CAD build for the part. Positions are in the model's coordinates, mm. A direction names the side the tool comes from. Round coordinates to 2 decimals unless told otherwise and drop trailing zeros. Order: outer loops, then holes, each group sorted by start corner. A loop starts at its lowest first (then second) coordinate and runs counter-clockwise, first axis right, second up. Notation, with made-up numbers: (-25.75, 42.5) - (23.25, 42.5) arc R29 cw to (23.25, 62.5) - close; hole circle Ø2 at (-14.75, 84). An arc over 180 degrees is marked (long way). Write item = value, one per line.
Autodesk Fusion 360 part; units mm, degrees
sketch "Sketch1" plane through (0, 0, 0) normal (0, 0, 1) x (1, 0, 0)
  circle A0 centre (0, 0) radius 115
  circle A1 centre (0, 0) radius 87.5 construction
  circle A2 centre (0, 0) radius 65
  circle A3 centre (0, 0) radius 50
  dimension "d1" = 230
  dimension "d2" = 175
  dimension "d3" = 130
  dimension "d4" = 100
extrude "Extrude1" add sketch "Sketch1" along normal blind 15 contours A0
extrude "Extrude2" add sketch "Sketch1" along normal blind 80 contours A2
sketch "Sketch2" plane through (0, 0, 15) normal (0, 0, 1) x (-1, 0, 0)
  circle A0 centre (0, 0) radius 65
  circle A1 centre (0, 0) radius 115
  circle A2 centre (0, 0) radius 87.5
  line L0 (0, 0) -> (0, -122.0079) construction
  line L1 (0, 0) -> (50.2765, -121.3782) construction
  circle A3 centre (33.4848, -80.8395) radius 7.5
  dimension "d11" = 22.5
  dimension "d12" = 15
extrude "Extrude3" cut sketch "Sketch2" along normal through all contours A2 A3 | A2 A3 picked at (32.6894, -78.4443) picked at (34.4384, -83.1246)
pattern_circular "C-Pattern1" count 8 over 360 about axis through (0, 0, 0) along (0, 0, 1) of "Extrude3"
(1) Probe line 1 along Y through (x, z) = (0, 56); line 2 along Z through (x, y) = (-12.5, -84); line 3 along X through (y, z) = (10, 17). List the from-to ranges inside material, lowest first.
Solved:
line_1 = -65 to -50, 50 to 65
line_2 = 0 to 15
line_3 = -64.23 to -48.99, 48.99 to 64.23
(2) Pull direction X, two halves, no side cores. Call faces 1 (the flat face through (33, -38, 80)), 2 (the cylindrical face through (47.69, -15.02, 39.44)), 3 (the cylindrical face through (-24.93, 112.265, 7.395)): released by +X, released by -X, zero draft, split by the parting line, or undercut.
Solved:
face_1 = zero draft
face_2 = undercut
face_3 = split by the parting line
(3) Drop flat-ended pins along their axis: pin 1 (1 mm diameter, centred on x = 26.5, y = -81, fed in from +Z); pin 2 (6 mm diameter, centred on y = -48.5, z = 21.5, fed in from +X); pin 3 (10 mm diameter, centred on y = 21, z = 8.5, fed in from -X). Give the stop position or say it passes through.
Solved:
pin_1 = 15
pin_2 = 46.42
pin_3 = -113.88
(4) Band-saw the part on A-A on y = 0. List the corners of the cut face in (x, z), plus the area to 3 significant figures.
Solved:
outline = (-115, 0) - (-50, 0) - (-50, 80) - (-65, 80) - (-65, 15) - (-115, 15) - close; (50, 0) - (115, 0) - (115, 15) - (65, 15) - (65, 80) - (50, 80) - close
area = 3,900 mm²
(5) Band-saw the part on C-C on z = 24. List the corners of the cut face in (x, y), plus the area to 3 significant figures.
Solved:
outline = circle Ø130 at (0, 0); hole circle Ø100 at (0, 0)
area = 5,420 mm²
(6) Band-saw the part on D-D on x = 96. List the corners of the cut face in (y, z).
Solved:
outline = (-63.32, 0) - (63.32, 0) - (63.32, 15) - (-63.32, 15) - close
(7) Tool access for faces 4 (the flat face through (24, -50, 0)), 5 (the flat face through (50, -50, 15)): list every direction of +Z, -Z, +X, -X, +Y, -Y with a clear straight run to the whole face (end or side of a thin tool).
Solved:
face_4 = -Z, +X, -X, +Y, -Y
face_5 = +Z
